Geometry: final body of the model. Coordinates: model frame, mm. Face numbers are marked on the shaded views. A direction names the side the tool comes from. Give positions to 0.01 mm unless a question says otherwise; leave off trailing zeros. Loops run counter-clockwise (first coordinate to the right, second up) from the corner with the lowest first, then second, coordinate; pieces in that order, holes last.
Autodesk Inventor part; units mm, degrees
ref_plane "YZ Plane" through (0, 0, 0) normal (1, 0, 0) x (0, 1, 0)
ref_plane "XZ Plane" through (0, 0, 0) normal (0, 1, 0) x (-1, 0, 0)
ref_plane "XY Plane" through (0, 0, 0) normal (0, 0, 1) x (1, 0, 0)
sketch "Sketch1" plane through (0, 0, 0) normal (1, 0, 0) x (0, 1, 0)
  line L0 (0, 0) -> (9.144, 0)
  line L1 (9.144, 0) -> (9.144, -25.4)
  line L2 (9.144, -25.4) -> (0, -25.4)
  line L3 (0, -25.4) -> (0, 0)
  dimension "d0" = 25.4
  dimension "d1" = 9.144
extrude "Extrusion1" add sketch "Sketch1" along normal blind 63.5
sketch "Sketch2" plane through (0, 9.144, 0) normal (0, 1, 0) x (1, 0, 0)
  line L0 (0, 25.4) -> (0, 0)
  line L1 (0, 12.7) -> (6.35, 12.7)
  line L2 (6.35, 12.7) -> (31.75, 12.7)
  line L3 (31.75, 12.7) -> (57.15, 12.7)
  circle A0 centre (6.35, 12.7) radius 4.7625
  circle A1 centre (31.75, 12.7) radius 4.7625
  circle A2 centre (57.15, 12.7) radius 4.7625
  dimension "d4" = 6.35
  dimension "d5" = 25.4
  dimension "d6" = 25.4
  dimension "d7" = 9.525
  dimension "d8" = 9.525
  dimension "d9" = 9.525
sketch "Sketch3" plane through (0, 0, 0) normal (-1, 0, 0) x (0, 0, 1)
  line L0 (-25.4, 0) -> (-25.4, 9.144)
  line L1 (0, 0) -> (-25.4, 0)
  line L2 (-25.4, 0) -> (-25.4, 9.144)
  line L3 (-25.4, 9.144) -> (0, 9.144)
  line L4 (0, 9.144) -> (0, 0)
extrude "Extrusion2" add sketch "Sketch3" along normal blind 3.175
extrude "Extrusion3" cut sketch "Sketch2" against normal blind 25.4
sketch "Sketch4" plane through (63.5, 0, 0) normal (1, 0, 0) x (0, 0, -1)
  line L0 (25.4, 0) -> (25.4, 9.144)
  line L1 (25.4, 9.144) -> (0, 9.144)
  line L2 (0, 9.144) -> (0, 0)
  line L3 (0, 0) -> (25.4, 0)
extrude "Extrusion4" add sketch "Sketch4" along normal blind 5.08
sketch "Sketch5" plane through (68.58, 0, 0) normal (1, 0, 0) x (0, 0, -1)
  line L0 (25.4, 9.144) -> (0, 9.144)
  line L1 (0, 9.144) -> (0, 0)
  line L2 (0, 0) -> (25.4, 0)
  line L3 (25.4, 0) -> (25.4, 9.144)
extrude "Extrusion5" add sketch "Sketch5" along normal blind 1.27
sketch "Sketch8" plane through (-3.175, 0, -25.4) normal (0, 0, -1) x (-1, 0, 0)
  line L0 (-73.025, 0) -> (0, 0)
  line L1 (0, 9.144) -> (-73.025, 9.144)
  line L2 (0, 0) -> (-15.875, 0)
  line L3 (-15.875, 0) -> (-15.875, 9.144)
  line L4 (-15.875, 9.144) -> (0, 9.144)
  line L5 (0, 9.144) -> (0, 0)
  line L6 (0, 9.144) -> (0, 0)
  point P0 (-3.175, 0)
  point P1 (0, 4.572)
  dimension "d24" = 15.875
extrude "Extrusion8" add sketch "Sketch8" along normal blind 50.8
sketch "Sketch9" plane through (-3.175, 0, 0) normal (-1, 0, 0) x (0, 0, 1)
  line L0 (0, 0) -> (0, 9.144)
  line L1 (0, 9.144) -> (-76.2, 9.144)
  line L2 (-76.2, 0) -> (-76.2, 9.144)
  line L3 (0, 0) -> (-76.2, 0)
extrude "Extrusion9" add sketch "Sketch9" along normal blind 3.175
sketch "Sketch10" plane through (69.85, 9.144, 0) normal (0, 1, 0) x (1, 0, 0)
  line L0 (-57.15, 25.4) -> (-57.15, 76.2)
  line L1 (-57.15, 76.2) -> (-66.675, 76.2)
  line L2 (-57.15, 76.2) -> (-76.2, 76.2)
  line L3 (-71.4375, 41.2761) -> (-61.9125, 41.2761)
  line L4 (-71.4375, 60.3261) -> (-61.9125, 60.3261)
  circle A0 centre (-66.675, 41.2761) radius 4.7625
  circle A1 centre (-66.675, 60.3261) radius 4.7625
  line L5 (-71.4375, 41.2761) -> (-71.4375, 60.3261)
  line L6 (-61.9125, 60.3261) -> (-61.9125, 41.2761)
  point P0 (-69.85, 0)
  dimension "d55" = 9.525
  dimension "d29" = 9.525
  dimension "d56" = 9.525
extrude "Extrusion10" add sketch "Sketch10" along normal blind 35.179
sketch "Sketch11" plane through (-3.175, 0, -76.2) normal (0, 0, -1) x (-1, 0, 0)
  line L0 (-15.875, 9.144) -> (3.175, 9.144)
  line L1 (-15.875, 9.144) -> (-15.875, 0)
  line L2 (-15.875, 0) -> (3.175, 0)
  line L3 (3.175, 9.144) -> (3.175, 0)
  point P0 (-3.175, 0)
extrude "Extrusion11" add sketch "Sketch11" along normal blind 25.4
sketch "Sketch13" plane through (12.7, 0, -25.4) normal (1, 0, 0) x (0, 0, -1)
  line L0 (0, 9.144) -> (76.2, 9.144)
  line L1 (-25.4, 0) -> (76.2, 0)
  line L2 (76.2, 9.144) -> (50.8, 9.144)
  line L3 (50.8, 9.144) -> (50.8, 0)
  line L4 (50.8, 0) -> (76.2, 0)
  line L5 (76.2, 0) -> (76.2, 9.144)
  dimension "d38" = 25.4
extrude "Extrusion12" add sketch "Sketch13" along normal blind 57.15
sketch "Sketch14" plane through (69.85, 9.144, 0) normal (0, 1, 0) x (1, 0, 0)
  circle A0 centre (-12.7, 12.7) radius 4.7625
  line L0 (-12.7, 12.7) -> (-12.7, 88.9)
  circle A1 centre (-38.1, 12.7) radius 4.7625
  line L1 (-38.1, 12.7) -> (-38.1, 88.9)
  circle A2 centre (-12.7, 88.9) radius 4.7625
  circle A3 centre (-38.1, 88.9) radius 4.7625
  circle A4 centre (-63.5, 12.7) radius 4.7625
  line L2 (-63.5, 12.7) -> (-63.5, 88.9)
  circle A5 centre (-63.5, 88.9) radius 4.7625
  point P0 (-69.85, 0)
  dimension "d42" = 76.2
  dimension "d43" = 76.2
  dimension "d44" = 9.525
  dimension "d45" = 9.525
  dimension "d46" = 9.525
extrude "Extrusion13" cut sketch "Sketch14" against normal blind 20.6375 contours A2 | A3 | A5
fillet "Fillet2" radius 7.9375 2 edges at (-6.35, 4.572, -101.6) (-6.35, 4.572, 0)
sketch "Sketch15" plane through (69.85, 9.144, 0) normal (0, 1, 0) x (1, 0, 0)
  line L0 (0, 25.4) -> (-57.15, 25.4)
  line L1 (-57.15, 25.4) -> (-76.2, 25.4)
  line L2 (-76.2, 7.9375) -> (-76.2, 93.6625)
  line L3 (-57.15, 25.4) -> (-57.15, 76.2)
  line L4 (-57.15, 76.2) -> (-76.2, 76.2)
  line L5 (-71.4375, 31.7511) -> (-71.4375, 69.8511)
  line L6 (-61.9125, 69.8511) -> (-61.9125, 31.7511)
  arc A0 (-71.4375, 31.7511) -> (-61.9125, 31.7511) centre (-66.675, 31.7511) ccw
  arc A1 (-61.9125, 69.8511) -> (-71.4375, 69.8511) centre (-66.675, 69.8511) ccw
  arc A2 (-71.4375, 41.2761) -> (-61.9125, 41.2761) centre (-66.675, 41.2761) ccw
  arc A3 (-61.9125, 60.3261) -> (-71.4375, 60.3261) centre (-66.675, 60.3261) ccw
  point P0 (-69.85, 0)
extrude "Extrusion14" add sketch "Sketch15" along normal blind 26.035 contours L1 L2 L4 L3 | L5 A2 L6 A0 | L5 A1 L6 A3
fillet "Fillet3" radius 6.35 2 edges at (3.175, 35.179, -76.2) (3.175, 35.179, -25.4)
sketch "Sketch16" plane through (-1.5875, 44.323, -60.3261) normal (-1, 0, 0) x (0, 0, 1)
  arc A0 (-9.5239, -9.144) -> (-15.8739, -15.494) centre (-9.5239, -15.494) ccw
  line L0 (-9.5239, -9.144) -> (49.3517, -9.144)
  line L1 (49.3517, -9.144) -> (49.3517, 6.1013)
  line L2 (49.3517, 6.1013) -> (-9.5239, 6.1013)
  line L3 (-9.5239, 6.1013) -> (-9.5239, -9.144)
  point P0 (60.3261, -44.323)
extrude "Extrusion15" cut sketch "Sketch16" against normal blind 21.971
sketch "Sketch19" plane through (69.85, 35.179, 0) normal (0, 1, 0) x (1, 0, 0)
  line L0 (-57.15, 76.2) -> (-76.2, 76.2)
  line L1 (-57.15, 25.4) -> (-76.2, 25.4)
  line L2 (-57.15, 76.2) -> (-66.675, 76.2)
  line L3 (-66.675, 76.2) -> (-66.675, 25.4)
  line L4 (-66.675, 25.4) -> (-57.15, 25.4)
  line L5 (-57.15, 25.4) -> (-57.15, 76.2)
  line L6 (-57.15, 76.2) -> (-49.094, 76.2)
  line L7 (-49.094, 76.2) -> (-49.094, 25.4)
  line L8 (-49.094, 25.4) -> (-57.15, 25.4)
  line L9 (-57.15, 25.4) -> (-57.15, 76.2)
  point P0 (-69.85, 0)
extrude "Extrusion18" cut sketch "Sketch19" against normal blind 42.8625
fillet "Fillet8" radius 6.35 2 edges at (3.175, 4.572, -76.2) (3.175, 4.572, -25.4)
properties part number "CH-1-03-RearGearboxSpacer_01"
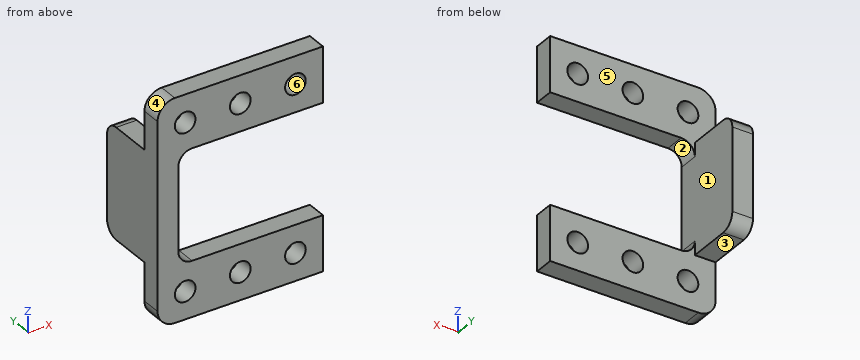
Item 1: Section query B-B on x = 39.5. Return loops of the section in (y, z), plus the area to 3 significant figures.
Values follow:
outline: (0, -101.6) - (9.14, -101.6) - (9.14, -76.2) - (0, -76.2) - close; (0, -25.4) - (9.14, -25.4) - (9.14, 0) - (0, 0) - close
area: 465 mm2
Item 2: Section query A-A on z = -12.7. Return loops of the section in (x, y), plus the area to 3 significant figures.
Values follow:
outline: (-6.35, 0) - (1.59, 0) - (1.59, 9.14) - (-6.35, 9.14) - close; (11.11, 0) - (26.99, 0) - (26.99, 9.14) - (11.11, 9.14) - close; (36.51, 0) - (52.39, 0) - (52.39, 9.14) - (36.51, 9.14) - close; (61.91, 0) - (69.85, 0) - (69.85, 9.14) - (61.91, 9.14) - close
area: 435 mm2
Item 3: Draft query along Z for the marked faces 4, 5 and 6. Return one class per face: +Z half, -Z half, draft (parallel to the pull), parting line (faces both ways), or undercut.
Values follow:
face 4: +Z half
face 5: draft
face 6: undercut
Item 4: Pin query (flat end, axial travel): pin 1 (5.5 mm diameter, centred on x = 6.35, z = -12.7, fed in from -Y); pin 2 (3 mm diameter, centred on x = 57.5, z = -75.5, fed in from +Y); pin 3 (5 mm diameter, centred on x = -2, y = 18.5, fed in from -Z); pin 4 (3 mm diameter, centred on x = -0.5, y = 19, fed in from +Z). Return the tip coordinate at first contact, or that it passes through.
Values follow:
pin 1: passes through
pin 2: stops at y = 9.14
pin 3: stops at z = -76.2
pin 4: stops at z = -25.4
Item 5: Section query D-D on z = -83. Return loops of the section in (x, y), plus the area to 3 significant figures.
Values follow:
outline: (-6.35, 0) - (69.85, 0) - (69.85, 9.14) - (-6.35, 9.14) - close
area: 697 mm2
Item 6: Set-up query: the marked faces 1, 2 and 3. Return all of +Z, -Z, +X, -X, +Y, -Y with unobstructed straight access to the full face (end or side cutting, diameter ignored); none if empty.
Values follow:
face 1: +X, +Y
face 2: +X, +Y, -Y
face 3: -Z, +X, -X, +Y
Item 7: Ray query, probe 1 along Z at (x, y) = (31.75, 4.75); probe 2 along X at (y, z) = (2.75, -12.7); probe 3 along Z at (x, y) = (31, 2). Return the intervals inside material, ascending.
Values follow:
probe 1: z = -101.6 to -93.66, -84.14 to -76.2, -25.4 to -17.46, -7.94 to 0
probe 2: x = -6.35 to 1.59, 11.11 to 26.99, 36.51 to 52.39, 61.91 to 69.85
probe 3: z = -101.6 to -93.6, -84.2 to -76.2, -25.4 to -17.4, -8 to 0
Item 8: Section query C-C on x = 57.15. Return loops of the section in (y, z), plus the area to 3 significant figures.
Values follow:
outline: (0, -101.6) - (9.14, -101.6) - (9.14, -93.66) - (0, -93.66) - close; (0, -84.14) - (9.14, -84.14) - (9.14, -76.2) - (0, -76.2) - close; (0, -25.4) - (9.14, -25.4) - (9.14, -17.46) - (0, -17.46) - close; (0, -7.94) - (9.14, -7.94) - (9.14, 0) - (0, 0) - close
area: 290 mm2
